Input: part model. Units: mm. Frame: model coordinates. Give positions to 0.01 mm unless a question says otherwise; leave off trailing zeros. Loops run counter-clockwise (first coordinate to the right, second up) from the corner with the lowest first, then second, coordinate; pieces in that order, holes last. Notation, with made-up numbers: (8, 76) - (34, 76) arc R26 cw to (34, 99) - close; hole circle Ø7 at (-2, 14). An arc over 180 degrees is marked (long way). One line per item, written item: value.
from build123d import *

# Parameters (mm, degrees)
F1_W     = 127
F1_H     = 127
F2_DEPTH = 5
F5_R     = 2.5


with BuildPart() as f2:
    # F1 (on Top) → F2 (new body)
    with BuildSketch(Plane.XY):
        Rectangle(F1_W, F1_H)
    extrude(amount=F2_DEPTH)

    # F3 (on Front) → F4 (revolve)
    with BuildSketch(Plane.XZ):
        with BuildLine():
            Line((-5.3333333333, 5), (0, 5))
            Line((0, 5), (0, 35))
            add(Edge.make_bspline(
                [(0, 35), (-6.5041498378, 34.8856949083), (-11.8426118801, 27.7496803572), (-10.0399512827, 13.5458032148), (-4.8367147753, 9.4293111278), (-5.3333333333, 5)],
                knots=[0, 0, 0, 0, 0.3484232949, 0.6924985169, 1, 1, 1, 1], degree=3))
        make_face()
    revolve(axis=Axis((0, 0, 20), (0, 0, 1)))

    # F5
    f5_edges = [f2.edges().sort_by_distance(p)[0] for p in [
        (0, -63.5, 5),
        (-63.5, 0, 5),
        (63.5, 0, 5),
        (0, 63.5, 5),
        (5.333333, 0, 5),
    ]]
    fillet(f5_edges, radius=F5_R)


solid = f2.part
Item 1: Pin query (flat end, axial travel): P1, Ø10, axis at x = -42.5, y = 33.5, coming from the +Z side; P2, Ø12, axis at y = 10.5, z = 9.5, coming from the -X side. Return the tip coordinate at first contact, or that it passes through.
Verdict:
P1: stops at z = 5
P2: stops at x = -63.29
Item 2: Material intervals for L1, parallel to Z at x = -31.5, y = -24.5; L2, parallel to X at y = -6, z = 29.5; L3, parallel to X at y = -4.5, z = 13, sorted ascending.
Verdict:
L1: z = 0 to 5
L2: x = -7.2 to 7.2
L3: x = -6.64 to 6.64
Item 3: Section A-A, the plane x = -25. Output: boundary loops of the cut face in (y, z).
Verdict:
outline: (-63.5, 0) - (63.5, 0) - (63.5, 2.5) arc R2.5 ccw to (61, 5) - (-61, 5) arc R2.5 ccw to (-63.5, 2.5) - close
